Here's how the part is built. I have some questions about the finished solid (model axes, mm). A direction names the side the tool comes from. Coordinates: 2 decimals unless noted, no trailing zeros. Write each loop counter-clockwise with the first axis right and the second up, starting at its lowest first coordinate (ties: lowest second). Pieces come first, ordered by that corner, then holes. Notation, with made-up numbers: (7.25, 60.5) - (16.25, 60.5) arc R14 cw to (16.25, 86.5) - close; hole circle Ø4 at (-34, 21). An arc over 180 degrees is marked (long way). Answer in a Markdown table with one row per item. Add a question column.
Item 1: If I drill on probe 1 along Y at (x, z) = (-1.75, 4.5); probe 2 along Y at (x, z) = (-3.75, 7.5); probe 3 along Y at (x, z) = (0, -1.35), over which ranges is the centre line in solid material (lowest first)? Write a range as from..to.
Item 2: I'm going to push flat-ended pins straight in: pin 1 (6 mm diameter, centred on y = -23.5, z = 4, fed in from -X); pin 2 (3 mm diameter, centred on x = -0.5, y = 6.5, fed in from -Z); pin 3 (2 mm diameter, centred on y = -24.257, z = 4.445, fed in from +X); pin 4 (2.5 mm diameter, centred on x = 0, y = 0, fed in from +Z). Where does each tip first touch, or does it pass through?
Item 3: Imagine slicing it at D-D (z = 5). Please give me the cut outline in (x, y), plus the area to 3 significant figures.
Item 4: Imagine slicing it at B-B (x = 0.25). Please give me the cut outline in (y, z) (3 decimals).
Item 5: Imagine slicing it at A-A (z = 1.75). Please give me the cut outline in (x, y).
Item 6: Which directions (+Z, -Z, +X, -X, +Y, -Y) give clear straight access to the entire face, cutting with the end or side of a thin tool? Please do faces 5 (the face through (1, -20.447, 5)), 6 (the face through (-2.606, 6.975, -3.828)), 7 (the face through (-5.08, 23, 6)).
Item 7: We'd pull the mould along Y, two halves only. Please class faces 1 (the face through (0, 27.94, 2)), 2 (the face through (-2, 0, 0)), 3 (the face through (0, -27.94, 2)), 4 (the face through (-7.62, 0, -3)): +Y half, -Y half, draft (parallel to the pull), parting line (faces both ways), or undercut.
Item 8: Imagine slicing it at C-C (x = 3.75). Please give me the cut outline in (y, z) (3 decimals).
from build123d import *

# Parameters (mm, degrees)
F1_DEPTH  = 7.62
F3_R      = 1.651
F4_DEPTH  = 25.4
F6_DEPTH  = 2.54
F8_D      = 2.032
F9_W      = 7.493
F9_H      = 9.525
F9_R      = 1.651
F10_DEPTH = 2.54


with BuildPart() as f1:
    # F0 (on Right) → F1 (new body, symmetric)
    with BuildSketch(Plane.YZ):
        Polygon((0, 0), (0, -5.08), (27.94, -5.08), (27.94, 9.525), (20.447, 9.525), (20.447, 0), align=None)
    extrude(amount=F1_DEPTH, both=True)

    # F2: F1 across plane


with BuildPart() as f1_1:
    add(f1.part)
    add(f1.part.mirror(Plane.XZ))

    # F3 (on face) → F4 (cut)
    with BuildSketch(Plane.YZ.offset(7.62)):
        with Locations((-24.257, 4.445)):
            Circle(F3_R)
        with Locations((24.257, 4.445)):
            Circle(F3_R)
    extrude(amount=-F4_DEPTH, mode=Mode.SUBTRACT)

    # F5 (on face) → F6 (cut)
    with BuildSketch(Plane(origin=(0, 0, -5.08), x_dir=(1, 0, 0), z_dir=(0, 0, -1))):
        with BuildLine():
            Line((-3.164081, -0.263095), (-2.032, -13.877949))
            ThreePointArc((-2.032, -13.877949), (0, -15.748), (2.032, -13.877949))
            Line((2.032, -13.877949), (3.164081, -0.263095))
            ThreePointArc((3.164081, -0.263095), (3.175, 0), (3.164081, 0.263095))
            Line((3.164081, 0.263095), (2.032, 13.877949))
            ThreePointArc((2.032, 13.877949), (0, 15.748), (-2.032, 13.877949))
            Line((-2.032, 13.877949), (-3.164081, 0.263095))
            ThreePointArc((-3.164081, 0.263095), (-3.175, 0), (-3.164081, -0.263095))
        make_face()
    extrude(amount=-F6_DEPTH, mode=Mode.SUBTRACT)

    # F8 (through all)
    with Locations(Plane(origin=(0, 0, -2.54), x_dir=(1, 0, 0), z_dir=(0, 0, -1))):
        with Locations((0, 0)):
            Hole(F8_D / 2)

    # F9 (on face) → F10 (cut)
    with BuildSketch(Plane(origin=(-7.62, 0, 0), x_dir=(0, -1, 0), z_dir=(-1, 0, 0))):
        with Locations((-24.1935, 4.7625)):
            Rectangle(F9_W, F9_H)
        with Locations((-24.257, 4.445)):
            Circle(F9_R, mode=Mode.SUBTRACT)
        with Locations((24.1935, 4.7625)):
            Rectangle(F9_W, F9_H)
        with Locations((24.257, 4.445)):
            Circle(F9_R, mode=Mode.SUBTRACT)
    extrude(amount=-F10_DEPTH, mode=Mode.SUBTRACT)


solid = f1_1.part
Here are the results:
| question | item | result |
|---|---|---|
| 1 | probe 1 | y = -27.94..-25.91, -22.61..-20.45, 20.45..22.61, 25.91..27.94 |
| 1 | probe 2 | y = -27.94..-20.45, 20.45..27.94 |
| 1 | probe 3 | y = -27.94..-1.02, 1.02..27.94 |
| 2 | pin 1 | stops at x = -5.08 |
| 2 | pin 2 | stops at z = -2.54 |
| 2 | pin 3 | passes through |
| 2 | pin 4 | stops at z = 0 |
| 3 | outline | (-5.08, -27.94) - (7.62, -27.94) - (7.62, -25.81) - (-5.08, -25.81) - close; (-5.08, -22.7) - (7.62, -22.7) - (7.62, -20.45) - (-5.08, -20.45) - close; (-5.08, 20.45) - (7.62, 20.45) - (7.62, 22.7) - (-5.08, 22.7) - close; (-5.08, 25.81) - (7.62, 25.81) - (7.62, 27.94) - (-5.08, 27.94) - close |
| 3 | area | 111 mm2 |
| 4 | outline | (-27.94, -5.08) - (-15.733, -5.08) - (-15.733, -2.54) - (-0.985, -2.54) - (-0.985, 0) - (-20.447, 0) - (-20.447, 9.525) - (-27.94, 9.525) - close; (0.985, -2.54) - (15.733, -2.54) - (15.733, -5.08) - (27.94, -5.08) - (27.94, 9.525) - (20.447, 9.525) - (20.447, 0) - (0.985, 0) - close; hole circle Ø3.302 at (-24.257, 4.445); hole circle Ø3.302 at (24.257, 4.445) |
| 5 | outline | (-5.08, -27.94) - (7.62, -27.94) - (7.62, -20.45) - (-5.08, -20.45) - close; (-5.08, 20.45) - (7.62, 20.45) - (7.62, 27.94) - (-5.08, 27.94) - close |
| 6 | face 5 | +Z, +X, -X |
| 6 | face 6 | -Z |
| 6 | face 7 | +Z, -X, +Y, -Y |
| 7 | face 1 | +Y half |
| 7 | face 2 | undercut |
| 7 | face 3 | -Y half |
| 7 | face 4 | draft |
| 8 | outline | (-27.94, -5.08) - (27.94, -5.08) - (27.94, 9.525) - (20.447, 9.525) - (20.447, 0) - (-20.447, 0) - (-20.447, 9.525) - (-27.94, 9.525) - close; hole circle Ø3.302 at (-24.257, 4.445); hole circle Ø3.302 at (24.257, 4.445) |
